Geometry check sheet. Reference: the model listing, model coordinates, mm. A direction names the side the tool comes from. Round coordinates to 2 decimals unless told otherwise and drop trailing zeros. Write each loop counter-clockwise with the first axis right and the second up, starting at its lowest first coordinate (ties: lowest second). Pieces come first, ordered by that corner, then holes. Notation, with made-up numbers: (-1, 75) -> (8, 75) arc R13 ccw to (8, 93) -> close; hole circle Ø9 at (-17, 31). An arc over 180 degrees is marked (long way). Put each result on its own line as item: value. Start each with the question number.
from build123d import *

# Parameters (mm, degrees)
SKETCH024_W             = 24
SKETCH024_H             = 10
SKETCH024_R             = 2.25
PAD008_DEPTH            = 8
PAD009_DEPTH            = 10
POCKET_DEPTH            = 4
SKETCH027_R             = 5
PAD010_DEPTH            = 2
PAD010_DEPTH_BACK       = 12
SKETCH028_R             = 4
PAD011_DEPTH            = 7
PAD011_DEPTH_BACK       = 21
SKETCH029_R             = 4
PAD012_DEPTH            = 7
POCKET001_DEPTH         = 4
SKETCH031_R             = 2.25
HOLE001_DEPTH           = 50
BODY003_PLACEMENT_ANGLE = 180


with BuildPart() as part:
    # Sketch024 → Pad008 (new body)
    with BuildSketch(Plane.XZ):
        with Locations((0, 44)):
            Rectangle(SKETCH024_W, SKETCH024_H)
        with Locations((-7, 44)):
            Circle(SKETCH024_R, mode=Mode.SUBTRACT)
        with Locations((7, 44)):
            Circle(SKETCH024_R, mode=Mode.SUBTRACT)
    extrude(amount=-PAD008_DEPTH)

    # Sketch025 (on Face1 of Pad008) → Pad009 (join)
    with BuildSketch(Plane(origin=(0, 0, 49), x_dir=(-1, 0, 0), z_dir=(0, 0, 1))):
        with BuildLine():
            Line((-10, 0), (-10, -8))
            Line((-11.55, -8), (-10, -8))
            ThreePointArc((-11.55, -8), (-13.28241, -8.717587), (-14, -10.449996))
            Line((-14, -10.449996), (-14.000017, -22))
            Line((-22.000017, -22), (-14.000017, -22))
            Line((-22, -8), (-22.000017, -22))
            ThreePointArc((-14, 0), (-19.656854, -2.343146), (-22, -8))
            Line((-10, 0), (-14, 0))
        make_face()
        with BuildLine():
            Line((10, -8), (10, 0))
            Line((10, 0), (14, 0))
            ThreePointArc((22, -8), (19.656854, -2.343146), (14, 0))
            Line((22, -8), (22, -22))
            Line((14, -22), (22, -22))
            Line((14, -10.45), (14, -22))
            ThreePointArc((14, -10.45), (13.282412, -8.717588), (11.55, -8))
            Line((10, -8), (11.55, -8))
        make_face()
    extrude(amount=-PAD009_DEPTH)

    # Sketch026 (on Face10 of Pad009) → Pocket (cut)
    with BuildSketch(Plane(origin=(0, 8, 0), x_dir=(1, 0, 0), z_dir=(0, 1, 0))):
        Polygon((-3.535898, -46), (-3.535898, -42), (-7, -40), (-10.464102, -42), (-10.464102, -46), (-7, -48), align=None)
        Polygon((10.464102, -46), (10.464102, -42), (7, -40), (3.535898, -42), (3.535898, -46), (7, -48), align=None)
    extrude(amount=-POCKET_DEPTH, mode=Mode.SUBTRACT)

    # Sketch027 (on Face3 of Pocket) → Pad010 (join, two sides)
    with BuildSketch(Plane(origin=(0, 0, 49), x_dir=(-1, 0, 0), z_dir=(0, 0, 1))) as pad010_sk:
        with Locations((-18, -22)):
            Circle(SKETCH027_R)
        with Locations((18, -22)):
            Circle(SKETCH027_R)
    extrude(amount=PAD010_DEPTH)
    extrude(pad010_sk.sketch, amount=-PAD010_DEPTH_BACK)

    # Sketch028 (on Face36 of Pad010) → Pad011 (join, two sides)
    with BuildSketch(Plane(origin=(0, 0, 51), x_dir=(-1, 0, 0), z_dir=(0, 0, 1))) as pad011_sk:
        with Locations((-18, -22)):
            Circle(SKETCH028_R)
    extrude(amount=PAD011_DEPTH)
    extrude(pad011_sk.sketch, amount=-PAD011_DEPTH_BACK)

    # Sketch029 (on Face50 of Pad011) → Pad012 (join)
    with BuildSketch(Plane(origin=(0, 0, 51), x_dir=(-1, 0, 0), z_dir=(0, 0, 1))):
        with Locations((18, -22)):
            Circle(SKETCH029_R)
    extrude(amount=PAD012_DEPTH)

    # Sketch030 (on Face49 of Pad012) → Pocket001 (cut)
    with BuildSketch(Plane(origin=(0, 0, 37), x_dir=(1, 0, 0), z_dir=(0, 0, -1))):
        Polygon((-14.535898, -24), (-14.535898, -20), (-18, -18), (-21.464102, -20), (-21.464102, -24), (-18, -26), align=None)
    extrude(amount=-POCKET001_DEPTH, mode=Mode.SUBTRACT)

    # Sketch031 (on Face61 of Pocket001) → Hole001 (cut)
    with BuildSketch(Plane(origin=(0, 0, 58), x_dir=(-1, 0, 0), z_dir=(0, 0, 1))):
        with Locations((18, -22)):
            Circle(SKETCH031_R)
        with Locations((-18, -22)):
            Circle(SKETCH031_R)
    extrude(amount=-HOLE001_DEPTH, mode=Mode.SUBTRACT)


with BuildPart() as part_1:
    # Body003 placement: moved
    add(part.part.moved(Location((18, 169, -23))).rotate(Axis((18, 169, -23), (0, 0, 1)), BODY003_PLACEMENT_ANGLE))


solid = part_1.part
(1) Material ranges on L1, parallel to Y at x = 0, z = 13.75; L2, parallel to X at y = 147.75, z = 23; L3, parallel to X at y = 154, z = 18.75, recorded low to high. Write a range as from..to.
(2) Sectioned sample at A-A (z = 15.5). Record the cut outline in (x, y), and give its area (3 significant figures).
(3) Sectioned sample at D-D (y = 154.75). Record the cut outline in (x, z), and give its area (3 significant figures).
(4) Sectioned sample at C-C (x = 35). Record the cut outline in (y, z), and give its area (3 significant figures).
(5) Mould release check, pull along X, two halves, no side actions. Record for faces 1 (the flat face through (32.536, 147, 16)), 2 (the flat face through (40, 156, 21)), 3 (the flat face through (38, 145, 35)), 4 (the flat face through (18, 161, 21)): +X half, -X half, draft (parallel to the pull), parting line (faces both ways), or undercut.
(6) Sectioned sample at B-B (z = 21). State how many separate pieces and enclosed holes the cut face has, and give its area (3 significant figures).
(7) Go/stop test with flat-tipped pins: pin 1 Ø9.5 at (x, y) = (26, 158.5) entering from -Z; pin 2 Ø10 at (x, z) = (18.5, 19) entering from -Y; pin 3 Ø4.5 at (y, z) = (163, 20.5) entering from -X; pin 4 Ø3 at (x, y) = (0.5, 147) entering from +Z. Record where each tip stops, or that it passes through.
(8) Set-up check for faces 5 (the flat face through (37.708, 150.014, 15.972)), 6 (the cylindrical face through (-0.521, 150.966, 31.451)), 7 (the flat face through (28.464, 163, 21)), 8 (the flat face through (2, 145, 35)): record each of +Z, -Z, +X, -X, +Y, -Y from which the full face is reachable in a straight line by a thin tool's end or side.
Found:
1. L1: 143..144.75, 149.25..151
1. L2: -4.94..-2.12, 2.12..4.94, 31.06..33.88, 38.12..40.94
1. L3: -4..4, 32..40
2. outline: circle Ø10 at (0, 147); circle Ø10 at (36, 147); hole circle Ø4.5 at (0, 147); hole (32.54, 145) -> (36, 143) -> (39.46, 145) -> (39.46, 149) -> (36, 151) -> (32.54, 149) -> close
2. area: 99.6 mm2
3. outline: (-4, 16) -> (4, 16) -> (4, 26) -> (-4, 26) -> close; (32, 16) -> (40, 16) -> (40, 26) -> (32, 26) -> close
3. area: 160 mm2
4. outline: (142.1, 14) -> (143.58, 14) -> (143.58, 18) -> (144.98, 18) -> (144.98, 35) -> (143.13, 35) -> (143.13, 28) -> (142.1, 28) -> close; (149.02, 18) -> (150.42, 18) -> (150.42, 14) -> (151.9, 14) -> (151.9, 16) -> (168.42, 16) -> (168.42, 26) -> (151.9, 26) -> (151.9, 28) -> (150.87, 28) -> (150.87, 35) -> (149.02, 35) -> close
4. area: 261 mm2
5. face 1: undercut
5. face 2: +X half
5. face 3: draft
5. face 4: undercut
6. separate pieces: 3
6. enclosed holes: 2
6. area: 515 mm2
7. pin 1: z = 16
7. pin 2: y = 161
7. pin 3: x = -4
7. pin 4: through
8. face 5: -Z
8. face 6: +Z
8. face 7: -Y
8. face 8: +Z, +X, -X, +Y, -Y
